The listing builds one solid part. Answer for the finished solid, in the listing's coordinates (mm). A direction names the side the tool comes from. Coordinates: 2 decimals unless noted, no trailing zeros. Loops run counter-clockwise (first coordinate to the right, second up) from the corner with the lowest first, then second, coordinate; pieces in that order, holes last. Notation, with made-up numbers: M 46.25,25 L 97.25,25 A32 cw 97.25,55 Z; hole C -20.75,29 d10. An arc over 180 degrees is marked long. Answer as a JSON object with one key per item and string values. Group by question number.
1. A cutting plane is placed at B-B on y = 21. Give the vertices of the cut face in (x, z).
2. A cutting plane is placed at A-A on z = 69.5. Give the vertices of the cut face in (x, y), and give its area (3 significant figures).
3. Straight lines are drawn through the part: L1, parallel to Z at x = 14, y = 36; L2, parallel to Z at x = 6.5, y = 33; L3, parallel to X at y = 35, z = 12. For each, find the intervals that lie inside material, in ascending order.
4. For faces 1 (the face through (25.39, 19.39, 74.84)), 2 (the face through (13.5, 15.4, 68.58)), 3 (the face through (25.394, 18.771, 88.793)), 4 (the face through (25, 23, 68.58)), 5 (the face through (3, 9, 10.16)), determine the directions among +Z, -Z, +X, -X, +Y, -Y from which every point of the face is accessible in a straight line to the end or side of a thin tool.
5. A cutting plane is placed at C-C on x = 28. Give the vertices of the cut face in (y, z).
6. A cutting plane is placed at D-D on y = 9. Give the vertices of the cut face in (x, z).
7. Given pin 1 (4 mm diameter, centred on x = 24, z = 80.5, fed in from -Y); pin 2 (3 mm diameter, centred on x = 17, z = 73, fed in from -Y); pin 3 (5 mm diameter, centred on x = 13.5, z = 23, fed in from -Y), each flat-ended and moving along its own axis, determine where each tip first touches the part or whether it passes through.
from build123d import *

# Parameters (mm, degrees)
SKETCH1_W           = 38.1
SKETCH1_H           = 38.1
BOSS_EXTRUDE1_DEPTH = 10.16
SKETCH2_R           = 18.415
BOSS_EXTRUDE2_DEPTH = 38.1
SKETCH3_W           = 38.1
SKETCH3_H           = 38.1
BOSS_EXTRUDE3_DEPTH = 10.16
SKETCH4_R           = 6.35
BOSS_EXTRUDE4_DEPTH = 10.16
BOSS_EXTRUDE5_DEPTH = 12.7
SKETCH6_R           = 6.35
BOSS_EXTRUDE6_DEPTH = 15.24


with BuildPart() as part:
    # Sketch1 → Boss-Extrude1 (new body)
    with BuildSketch(Plane.XY):
        with Locations((19.05, 19.05)):
            Rectangle(SKETCH1_W, SKETCH1_H)
    extrude(amount=BOSS_EXTRUDE1_DEPTH)

    # Sketch2 → Boss-Extrude2 (add)
    with BuildSketch(Plane.XY.offset(10.16)):
        with Locations(Location((19.05, 19.05, 0), (0, 0, 180))):
            Circle(SKETCH2_R)
    extrude(amount=BOSS_EXTRUDE2_DEPTH)

    # Sketch3 → Boss-Extrude3 (add)
    with BuildSketch(Plane.XY.offset(48.26)):
        with Locations((19.05, 19.05)):
            Rectangle(SKETCH3_W, SKETCH3_H)
    extrude(amount=BOSS_EXTRUDE3_DEPTH)

    # Sketch4 → Boss-Extrude4 (add)
    with BuildSketch(Plane.XY.offset(58.42)):
        with Locations(Location((19.05, 19.05, 0), (0, 0, 180))):
            Circle(SKETCH4_R)
    extrude(amount=BOSS_EXTRUDE4_DEPTH)

    # Sketch5 → Boss-Extrude5 (add)
    with BuildSketch(Plane.XY.offset(68.58)):
        Polygon((25.164098612, 23.097361053), (18.601931816, 26.368645246), (12.487833204, 22.321284193), (12.935901388, 15.002638947), (19.498068184, 11.731354754), (25.612166796, 15.778715807), align=None)
    extrude(amount=BOSS_EXTRUDE5_DEPTH)

    # Sketch6 → Boss-Extrude6 (add)
    with BuildSketch(Plane.XY.offset(81.28)):
        with Locations(Location((19.05, 19.05, 0), (0, 0, 180))):
            Circle(SKETCH6_R)
    extrude(amount=BOSS_EXTRUDE6_DEPTH)


solid = part.part
From the geometry:
{
 "1": {"outline": "M 0,0 L 38.1,0 L 38.1,10.16 L 37.36,10.16 L 37.36,48.26 L 38.1,48.26 L 38.1,58.42 L 25.09,58.42 L 25.09,68.58 L 25.29,68.58 L 25.29,81.28 L 25.09,81.28 L 25.09,96.52 L 13.01,96.52 L 13.01,81.28 L 12.57,81.28 L 12.57,68.58 L 13.01,68.58 L 13.01,58.42 L 0,58.42 L 0,48.26 L 0.74,48.26 L 0.74,10.16 L 0,10.16 Z"},
 "2": {"outline": "M 12.49,22.32 L 12.94,15 L 19.5,11.73 L 25.61,15.78 L 25.16,23.1 L 18.6,26.37 Z", "area": "140 mm²"},
 "3": {"L1": "z = 0 to 58.42", "L2": "z = 0 to 10.16, 48.26 to 58.42", "L3": "x = 9.85 to 28.25"},
 "4": {"face 1": "+Z, +X, +Y", "face 2": "-X, -Y", "face 3": "+Z", "face 4": "+X, +Y", "face 5": "none"},
 "5": {"outline": "M 0,0 L 38.1,0 L 38.1,10.16 L 35.14,10.16 L 35.14,48.26 L 38.1,48.26 L 38.1,58.42 L 0,58.42 L 0,48.26 L 2.96,48.26 L 2.96,10.16 L 0,10.16 Z"},
 "6": {"outline": "M 0,0 L 38.1,0 L 38.1,10.16 L 34.48,10.16 L 34.48,48.26 L 38.1,48.26 L 38.1,58.42 L 0,58.42 L 0,48.26 L 3.62,48.26 L 3.62,10.16 L 0,10.16 Z"},
 "7": {"pin 1": "stops at y = 13.39", "pin 2": "stops at y = 12.23", "pin 3": "stops at y = 0.89"}
}
